from build123d import *

# Parameters (mm, degrees)
F0_R     = 2.38125
F0_R_2   = 1.5875
F1_DEPTH = 0.79375
F2_DEPTH = 7.9375
F3_W     = 4.7625
F3_H     = 0.79375
F4_DEPTH = 0.79375
F3_W_2   = 6.35
F6_R     = 1.5875
F7_DEPTH = 4.7625
F8_R     = 1.5875
F9_DEPTH = 4.7625


with BuildPart() as f1:
    # F0 (on Top) → F1 (new body)
    with BuildSketch(Plane.XY):
        Circle(F0_R)
        Circle(F0_R_2, mode=Mode.SUBTRACT)
    extrude(amount=F1_DEPTH)

    # F0 (on Top) → F2 (join)
    with BuildSketch(Plane.XY):
        Circle(F0_R_2)
    extrude(amount=F2_DEPTH)

    # F3 (on Front) → F4 (join, symmetric)
    with BuildSketch(Plane.XZ):
        Polygon((2.38125, 0), (0, 0), (-2.38125, 0), (-3.96875, -2.749630657), (0.79375, -2.749630657), align=None)
        with Locations((-1.5875, -3.146505657)):
            Rectangle(F3_W, F3_H)
    extrude(amount=F4_DEPTH, both=True)



with BuildPart() as f4:
    # F3 (on Front) → F4, piece 2 (new body, symmetric)
    with BuildSketch(Plane.XZ):
        with Locations((-2.38125, -7.115255657)):
            Rectangle(F3_W_2, F3_H)
        with BuildLine():
            Line((3.0388140303, -9.7571946873), (0.79375, -7.512130657))
            Line((0.79375, -7.512130657), (-5.55625, -7.512130657))
            Line((-5.55625, -7.512130657), (1.1789420908, -14.2473227478))
            ThreePointArc((1.1789420908, -14.2473227478), (1.0634268399, -11.5692186432), (3.0388140303, -9.7571946873))
        make_face()
        with BuildLine():
            Line((1.1789420908, -14.2473227478), (3.0388140303, -9.7571946873))
            ThreePointArc((3.0388140303, -9.7571946873), (1.0634268399, -11.5692186432), (1.1789420908, -14.2473227478))
        make_face()
        with BuildLine():
            ThreePointArc((7.1717443556, -12.7842385409), (5.872803552, -10.2227883869), (3.0388140303, -9.7571946873))
            Line((3.0388140303, -9.7571946873), (1.1789420908, -14.2473227478))
            ThreePointArc((1.1789420908, -14.2473227478), (4.7497725122, -15.8686466844), (7.1717443556, -12.7842385409))
        make_face()
    extrude(amount=F4_DEPTH, both=True)


with BuildPart() as f1_1:
    add(f1.part)

    add(f4.part)  # F5 merges F4
    # F3 (on Front) → F5 (revolve)
    with BuildSketch(Plane.XZ):
        Polygon((-3.96875, -3.543380657), (-3.96875, -2.749630657), (-5.55625, -2.749630657), (-5.55625, -3.543380657), (-7.14375, -3.543380657), (-7.14375, -5.130880657), (-5.55625, -5.130880657), (0.79375, -5.130880657), (0.79375, -3.543380657), align=None)
        with Locations((-1.5875, -3.146505657)):
            Rectangle(F3_W, F3_H)
    revolve(axis=Axis((-2.38125, 0, -5.130880657), (1, 0, 0)))

    # F6 (on face) → F7 (join)
    with BuildSketch(Plane.XZ.offset(0.79375)):
        with Locations((3.9967443556, -12.7842385409)):
            Circle(F6_R)
    extrude(amount=F7_DEPTH)

    # F8 (on face) → F9 (join)
    with BuildSketch(Plane(origin=(0, 0.79375, 0), x_dir=(-1, 0, 0), z_dir=(0, 1, 0))):
        with Locations((-3.9967443556, -12.7842385409)):
            Circle(F8_R)
    extrude(amount=F9_DEPTH)


solid = f1_1.part
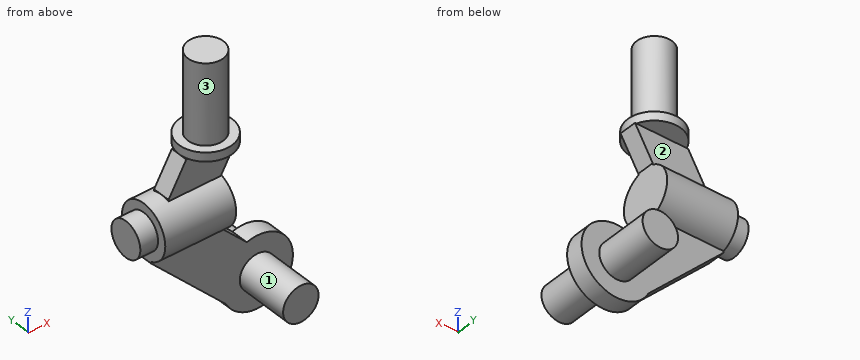
Work out the finished part from the listing and answer in its coordinate system (mm). Face numbers are marked on the shaded views. A direction names the side the tool comes from. Coordinates: 2 decimals unless noted, no trailing zeros. Write each loop counter-clockwise with the first axis right and the second up, starting at its lowest first coordinate (ties: lowest second). Pieces come first, ordered by that corner, then holes. Notation, with made-up numbers: M -24,59.25 L 33,59.25 A30 cw 33,88.25 Z; hole C 23.5,-34.5 d6. An arc over 180 degrees is marked long. Answer as CSV lines item,"result". Start each with the question number.
Item 1: Section C-C on y = 4.5 is taken. Write down the section's boundary in (x, z) (1 decimal), and give its area (3 significant figures).
Item 2: Section D-D on z = -2.5 is taken. Write down the section's boundary in (x, y).
Item 3: Consider L1, parallel to X at y = 0, z = -6; L2, parallel to Y at x = 1, z = -1; L3, parallel to X at y = 1.75, z = -5.5. Determine where each line is inside the solid, lowest interval first.
Item 4: A tool of negligible diameter and unlimited length cuts with its end or side. For the marked faces 1, 2 and 3, from which of +Z, -Z, +X, -X, +Y, -Y can it reach the whole face along a straight path? Write none if from no direction.
Item 5: Section A-A on x = 0.5 is taken. Write down the section's boundary in (y, z), and give its area (3 significant figures).
Item 6: Flat-ended cylindrical pins translate along their axes: P1, Ø2, axis at x = -5, z = -3.5, coming from the -Y side; P2, Ø8, axis at x = 3.5, z = -7, coming from the +Y side; P3, Ø1.3, axis at x = 0, y = -1.5, coming from the -Z side. Find the tip coordinate at first contact, or state that the pin passes through.
Item 7: Section B-B on z = -6 is taken. Write down the section's boundary in (x, y), and give its area (3 significant figures).
Checks:
1,outline,"C 4,-12.8 d3.2"
1,area,"7.92 mm²"
2,outline,"M -3.82,-0.79 L 0.94,-0.79 L 0.94,0.79 L -3.82,0.79 Z"
3,L1,"x = -7.14 to 0.79"
3,L2,"y = -0.79 to 0.79"
3,L3,"x = -5.56 to 0.79"
4,face 1,"-Y"
4,face 2,"+X, -X, +Y"
4,face 3,"+Z"
5,outline,"M -2.33,0 L -0.79,0 L -0.79,-2.89 A2.38 ccw -0.79,-7.38 L -0.79,-13.57 L 0.79,-13.57 L 0.79,-7.38 A2.38 ccw 0.79,-2.89 L 0.79,0 L 2.33,0 L 2.33,0.79 L 1.51,0.79 L 1.51,7.94 L -1.51,7.94 L -1.51,0.79 L -2.33,0.79 Z"
5,area,"57.2 mm²"
6,P1,"stops at y = -2.3"
6,P2,"stops at y = 2.38"
6,P3,"stops at z = -7.36"
7,outline,"M -7.14,-1.33 L -5.56,-1.33 L -5.56,-2.22 L 0.79,-2.22 L 0.79,2.22 L -5.56,2.22 L -5.56,1.33 L -7.14,1.33 Z"
7,area,"32.4 mm²"
